Could you check a few things on this model? Use its own coordinates, in mm. A direction names the side the tool comes from. Give positions to 0.01 mm unless a question says otherwise; leave off trailing zeros. Loops run counter-clockwise (first coordinate to the right, second up) from the corner with the lowest first, then second, coordinate; pieces in that order, holes last. Notation, with made-up numbers: M 20.5,85.25 L 41.5,85.25 A21 ccw 41.5,92.25 Z; hole C 11.5,77.5 d10. An arc over 180 degrees is marked long. Use a Markdown table: item, result. Add a question column.
1) Suppose I cut it at D-D on y = -6. List the corners of the cut face in (x, z) for me, and give its area (3 significant figures).
2) Will these pins go through, and if not, where does the flat tip stop? pin 1 Ø1.5 at (x, z) = (18.5, 79) entering from +Y; pin 2 Ø3.5 at (x, z) = (1, 16) entering from +Y; pin 3 Ø3 at (x, y) = (-1.5, 3.5) entering from -Z.
3) Which directions (+Z, -Z, +X, -X, +Y, -Y) give clear straight access to the entire face, cutting with the end or side of a thin tool? Please do faces 5 (the flat face through (15, 8, 63)), 6 (the flat face through (0, 5, 40.2)), 7 (the flat face through (13.5, -5, 63.4)), 8 (the flat face through (-16, 0, 63)).
4) Suppose I cut it at A-A on x = 0. List the corners of the cut face in (y, z) for me.
5) If I drill on line 1 along Z through (x, y) = (0, -7.5); line 2 along X through (y, z) = (2.05, 10); line 3 along X through (y, z) = (4.2, 115), over which ranges is the centre line in solid material (lowest first)? Write a range as [from, to].
6) We'd pull the mould along Z, two halves only. Please class faces 1 (the cylindrical face through (-0.16, -4.93, 28.86)), 2 (the cylindrical face through (0.577, -4.93, 11.209)), 3 (the flat face through (16, 0, 63)), 4 (the flat face through (0, -2, 0)): +Z half, -Z half, draft (parallel to the pull), parting line (faces both ways), or undercut.
7) Suppose I cut it at C-C on y = 2.75. List the corners of the cut face in (x, z) for me, and give its area (3 significant figures).
8) Suppose I cut it at B-B on z = 30.1. List the corners of the cut face in (x, y) for me, and give its area (4 significant figures).
Autodesk Inventor part; units mm, degrees
ref_plane "YZ Plane" through (0, 0, 0) normal (1, 0, 0) x (0, 1, 0)
ref_plane "XZ Plane" through (0, 0, 0) normal (0, 1, 0) x (-1, 0, 0)
ref_plane "XY Plane" through (0, 0, 0) normal (0, 0, 1) x (1, 0, 0)
sketch "Sketch1" plane through (0, 0, 0) normal (0, 0, 1) x (1, 0, 0)
  line L0 (-20, -10) -> (20, -10)
  line L1 (20, -10) -> (20, 10)
  line L2 (20, 10) -> (-20, 10)
  line L3 (-20, 10) -> (-20, -10)
  point P0 (0, 0)
  dimension "d0" = 40
  dimension "d1" = 20
  dimension "d2" = 10
  dimension "d3" = 20
extrude "Extrusion1" add sketch "Sketch1" along normal blind 125
sketch "Sketch2" plane through (-20, 10, 0) normal (0, 1, 0) x (1, 0, 0)
  line L0 (40, 0) -> (0, 0)
  line L1 (13.9, 0) -> (26.1, 0)
  line L2 (26.1, 0) -> (26.1, -40.2)
  line L3 (26.1, -40.2) -> (13.9, -40.2)
  line L4 (13.9, -40.2) -> (13.9, 0)
  point P0 (20, 0)
  point P1 (26.1, 0)
  dimension "d6" = 40.2
  dimension "d7" = 12.2
  dimension "d8" = 13.9
extrude "Extrusion2" cut sketch "Sketch2" against normal blind 10
sketch "Sketch3" plane through (-20, 10, 125) normal (0, 1, 0) x (1, 0, 0)
  line L0 (40, 125) -> (40, 0)
  line L1 (40, 125) -> (26.1, 125)
  line L2 (40, 0) -> (35, 0)
  line L3 (35, 0) -> (35, 125)
  line L4 (35, 125) -> (40, 125)
  line L5 (40, 125) -> (40, 0)
  point P0 (20, 125)
  dimension "d11" = 5
extrude "Extrusion3" cut sketch "Sketch3" against normal blind 4.3
sketch "Sketch4" plane through (-20, 0, 0) normal (0, 1, 0) x (1, 0, 0)
  circle A0 centre (20, -10.1) radius 1.25
  line L0 (13.9, 0) -> (26.1, 0)
  line L1 (13.9, -40.2) -> (13.9, 0)
  circle A1 centre (20, -30.1) radius 1.25
  point P0 (20, 0)
  dimension "d14" = 2.5
  dimension "d15" = 10.1
  dimension "d16" = 6.1
  dimension "d35" = 20
  dimension "d36" = 6.1
extrude "Extrusion4" cut sketch "Sketch4" against normal through all
sketch "Sketch5" plane through (0, 0, 125) normal (0, 0, 1) x (1, 0, 0)
  line L0 (-20, 10) -> (-20, -10)
  line L1 (20, -10) -> (20, 5.7)
  line L2 (-20, 0) -> (-10, 0)
  line L3 (-10, 0) -> (-20, -10)
  line L4 (-20, 0) -> (-20, -10)
  line L5 (20, 0) -> (20, -10)
  line L6 (20, 0) -> (10, 0)
  line L7 (10, 0) -> (20, -10)
  line L8 (-20, -10) -> (-17, -10)
  line L9 (-20, -10) -> (20, -10)
  line L10 (-10, 0) -> (-17, -10)
  line L11 (10, 0) -> (17, -10)
  line L12 (17, -10) -> (20, -10)
  point P0 (0, 0)
  dimension "d19" = 10
  dimension "d21" = 10
  dimension "d24" = 3
  dimension "d25" = 3
extrude "Extrusion5" cut sketch "Sketch5" against normal through all
fillet "Fillet1" radius 1 4 edges at (17, -10, 62.5) (10, 0, 62.5) (-17, -10, 62.5) (-10, 0, 62.5)
sketch "Sketch6" plane through (-20, 5.7, 125) normal (0, 1, 0) x (1, 0, 0)
  circle A0 centre (38.734, 10) radius 0.81
  circle A1 centre (38.734, 115) radius 0.81
  line L0 (40, 0) -> (35, 0)
  line L1 (35, 125) -> (40, 125)
  line L2 (35, 0) -> (35, 125)
  circle A2 centre (38.734, 62.5) radius 0.81
  point P0 (20, 125)
  dimension "d27" = 1.62
  dimension "d28" = 1.62
  dimension "d29" = 10
  dimension "d30" = 10
  dimension "d31" = 3.734
  dimension "d32" = 3.734
  dimension "d37" = 3.734
  dimension "d38" = 1.62
  dimension "d39" = 52.5
  dimension "d40" = 52.5
extrude "Extrusion6" cut sketch "Sketch6" against normal up to surface (5.7 mm away)
equation "\"d32\" = d31"
equation "\"d37\" = d31"
equation "\"d38\" = d27"
properties part number "3102_Dovetail Slider_V1" material "Acetal Resin, White"
Answer block:
| question | item | result |
|---|---|---|
| 1 | outline | M -14.2,0 L 14.2,0 L 14.2,125 L -14.2,125 Z; hole C 0,10.1 d2.5; hole C 0,30.1 d2.5 |
| 1 | area | 3,540 mm^2 |
| 2 | pin 1 | stops at y = 5.7 |
| 2 | pin 2 | stops at y = 0 |
| 2 | pin 3 | stops at z = 40.2 |
| 3 | face 5 | +Z, -Z, +X, +Y |
| 3 | face 6 | -Z, +Y |
| 3 | face 7 | +Z, -Z, +X |
| 3 | face 8 | +Z, -Z, -X |
| 4 | outline | M -10,0 L 0,0 L 0,8.85 L -10,8.85 Z; M -10,11.35 L 0,11.35 L 0,28.85 L -10,28.85 Z; M -10,31.35 L 0,31.35 L 0,40.2 L 10,40.2 L 10,125 L -10,125 Z |
| 5 | line 1 | z = [0, 8.85], [11.35, 28.85], [31.35, 125] |
| 5 | line 2 | x = [-20, -6.1], [6.1, 17.92], [19.54, 20] |
| 5 | line 3 | x = [-20, 17.92], [19.54, 20] |
| 6 | face 1 | undercut |
| 6 | face 2 | undercut |
| 6 | face 3 | draft |
| 6 | face 4 | -Z half |
| 7 | outline | M -20,0 L -6.1,0 L -6.1,40.2 L 6.1,40.2 L 6.1,0 L 20,0 L 20,125 L -20,125 Z; hole C 18.73,10 d1.62; hole C 18.73,62.5 d1.62; hole C 18.73,115 d1.62 |
| 7 | area | 4,500 mm^2 |
| 8 | outline | M -20,0 L -11.92,0 A1 cw -11.1,-1.57 L -15.9,-8.43 A1 ccw -15.08,-10 L -1.25,-10 L -1.25,0 L -6.1,0 L -6.1,10 L -20,10 Z; M 1.25,-10 L 15.08,-10 A1 ccw 15.9,-8.43 L 11.1,-1.57 A1 cw 11.92,0 L 20,0 L 20,5.7 L 15,5.7 L 15,10 L 6.1,10 L 6.1,0 L 1.25,0 Z |
| 8 | area | 501.5 mm^2 |
